Study the drawing (mm; zero at the part's minimum x, y, z) and answer. Coordinates: 2 decimals unless noted, no trailing zeros. Order: outer loops, then holes, each group sorted by start corner. A loop starts at its lowest first (then second) coordinate and runs counter-clockwise, first axis right, second up.
1. The part is cut by section B-B, the plane y = 5.5. Give the vertices of the cut face in (x, z).
2. The part is cut by section C-C, the plane z = 1.25. Give the vertices of the cut face in (x, y).
3. Find the intervals of material crossed by probe 1 along Y at (x, z) = (21.17, 0.45); probe 2 along Y at (x, z) = (22.5, 0.6) (1 decimal); probe 3 along X at (y, z) = (6, 1) (1 decimal), in increasing order.
4. The part is cut by section A-A, the plane x = 2.5. Give the vertices of the cut face in (y, z).
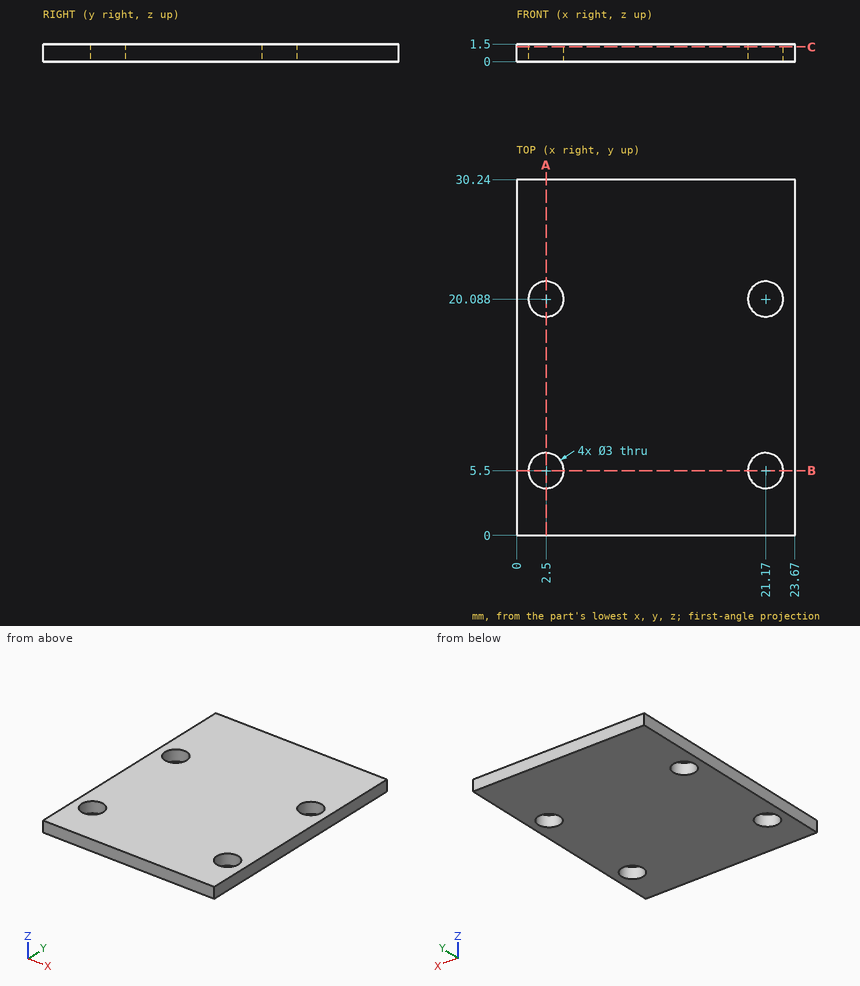
Geometry says:
1. outline: (0, 0) - (1, 0) - (1, 1.5) - (0, 1.5) - close; (4, 0) - (19.67, 0) - (19.67, 1.5) - (4, 1.5) - close; (22.67, 0) - (23.67, 0) - (23.67, 1.5) - (22.67, 1.5) - close
2. outline: (0, 0) - (23.67, 0) - (23.67, 30.24) - (0, 30.24) - close; hole circle Ø3 at (2.5, 5.5); hole circle Ø3 at (2.5, 20.09); hole circle Ø3 at (21.17, 5.5); hole circle Ø3 at (21.17, 20.09)
3. probe 1: y = 0 to 4, 7 to 18.59, 21.59 to 30.24
3. probe 2: y = 0 to 4.8, 6.2 to 19.4, 20.8 to 30.2
3. probe 3: x = 0 to 1.1, 3.9 to 19.8, 22.6 to 23.7
4. outline: (0, 0) - (4, 0) - (4, 1.5) - (0, 1.5) - close; (7, 0) - (18.59, 0) - (18.59, 1.5) - (7, 1.5) - close; (21.59, 0) - (30.24, 0) - (30.24, 1.5) - (21.59, 1.5) - close
